```python
from build123d import *

# Parameters (mm, degrees)
SKETCH1_W           = 40
SKETCH1_H           = 40
BOSS_EXTRUDE1_DEPTH = 3
SKETCH2_W           = 40
SKETCH2_H           = 3
BOSS_EXTRUDE2_DEPTH = 53
SKETCH3_W           = 40
SKETCH3_H           = 3
BOSS_EXTRUDE3_DEPTH = 20
CUT_EXTRUDE1_REACH  = 5
FILLET1_R           = 3
SKETCH5_W           = 40
SKETCH5_H           = 3
BOSS_EXTRUDE4_DEPTH = 20


with BuildPart() as part:
    # Sketch1 → Boss-Extrude1 (new body)
    with BuildSketch(Plane(origin=(0, 0, 0), x_dir=(1, 0, 0), z_dir=(0, 1, 0))):
        Rectangle(SKETCH1_W, SKETCH1_H)
    extrude(amount=BOSS_EXTRUDE1_DEPTH)

    # Sketch2 → Boss-Extrude2 (add)
    with BuildSketch(Plane(origin=(0, 0, 0), x_dir=(1, 0, 0), z_dir=(0, 1, 0))):
        with Locations((0, -21.5)):
            Rectangle(SKETCH2_W, SKETCH2_H)
    extrude(amount=BOSS_EXTRUDE2_DEPTH)

    # Sketch3 → Boss-Extrude3 (add)
    with BuildSketch(Plane.XZ):
        with Locations((0, -18.5)):
            Rectangle(SKETCH3_W, SKETCH3_H)
    extrude(amount=BOSS_EXTRUDE3_DEPTH)

    # Sketch4 → Cut-Extrude1 (cut, up to next)
    with BuildSketch(Plane(origin=(0, 0, 20), x_dir=(-1, 0, 0), z_dir=(0, 0, -1)), mode=Mode.PRIVATE) as cut_extrude1_sk1:
        with BuildLine():
            Line((-20, 37.641016151), (-20, 53))
            Line((-20, 53), (20, 53))
            Line((20, 53), (20, 37.641016151))
            ThreePointArc((20, 37.641016151), (0, 43), (-20, 37.641016151))
        make_face()
    cut_extrude1_tool1 = extrude(cut_extrude1_sk1.sketch, amount=-CUT_EXTRUDE1_REACH, mode=Mode.PRIVATE) & part.part
    add(cut_extrude1_tool1.solids().sort_by_distance((0, 47.025808, 20))[0], mode=Mode.SUBTRACT)

    # Fillet1
    fillet1_edges = [part.edges().sort_by_distance(p)[0] for p in [
        (0, 3, 20),
        (0, 3, -20),
    ]]
    fillet(fillet1_edges, radius=FILLET1_R)

    # Sketch5 → Boss-Extrude4 (add)
    with BuildSketch(Plane.XY.offset(-17)):
        with Locations((0, -18.5)):
            Rectangle(SKETCH5_W, SKETCH5_H)
    extrude(amount=BOSS_EXTRUDE4_DEPTH)


solid = part.part
```
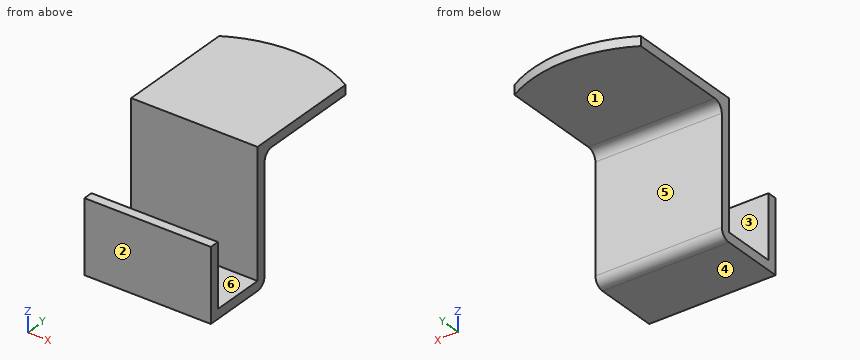
For this review, take the finished solid that the model builds, in its own axes (mm). Face numbers are marked on the shaded views. A direction names the side the tool comes from. Round coordinates to 2 decimals unless told otherwise and drop trailing zeros. Write each loop counter-clockwise with the first axis right and the second up, starting at its lowest first coordinate (ties: lowest second). Pieces come first, ordered by that corner, then holes. Notation, with made-up numbers: (68.25, -28) - (112.25, -28) arc R18 cw to (112.25, -14) - close; hole circle Ø7 at (52, 81.5). An arc over 180 degrees is marked (long way). Answer as CSV lines item,"result". Start each with the question number.
(1) Machinability: for the marked faces 1, 2 and 3, which of the approach directions +Z, -Z, +X, -X, +Y, -Y give a long, thin tool a straight path to every point of the face, cutting with its end or side? Answer none if there is none.
(2) For pin 1 (4 mm diameter, centred on x = 14, z = 12, fed in from +Y); pin 2 (13.5 mm diameter, centred on x = -7, y = -9.5, fed in from +Z); pin 3 (1 mm diameter, centred on x = 1.5, z = 17.5, fed in from -Y); pin 4 (12 mm diameter, centred on y = -4, z = 13, fed in from +X), all flat-tipped, find the tip position at first contact; note any pin that passes through.
(3) Add section A-A, the plane z = -10. State the section outline as (x, y) points.
(4) Add section D-D, the plane x = 7. State the section outline as (y, z) points, plus the area to 3 significant figures.
(5) Mouldability with a two-part tool opening along Y and no side actions: class the marked faces 4, 5 and 6 as +Y half, -Y half, draft (parallel to the pull), parting line (faces both ways), or undercut.
(6) For line 1 (Y direction, x = -9.5, z = 0); line 2 (Z direction, x = -4.5, y = -11); line 3 (Y direction, x = -12, z = 8), list the stretches that pass through material, from the lowest coordinate up.
(7) Add section C-C, the plane y = -11.5. State the section outline as (x, z) points.
(8) Add section B-B, the plane x = 0. State the section outline as (y, z) points, plus the area to 3 significant figures.
From the geometry:
1,face 1,"-Z, +X, -X, +Y"
1,face 2,"+Z, -Z, +X, -X, -Y"
1,face 3,"+Z, +X, -X"
2,pin 1,"stops at y = 3"
2,pin 2,"stops at z = -17"
2,pin 3,"stops at y = 0"
2,pin 4,"stops at x = 20"
3,outline,"(-20, -20) - (20, -20) - (20, -17) - (-20, -17) - close; (-20, 0) - (20, 0) - (20, 3) - (-20, 3) - close"
4,outline,"(-20, -20) - (0, -20) arc R3 ccw to (3, -17) - (3, 17) arc R3 cw to (6, 20) - (42.38, 20) - (42.38, 23) - (0, 23) - (0, -17) - (-17, -17) - (-17, 3) - (-20, 3) - close"
4,area,"367 mm²"
5,face 4,"draft"
5,face 5,"+Y half"
5,face 6,"undercut"
6,line 1,"y = -20 to -17, 0 to 3"
6,line 2,"z = -20 to -17"
6,line 3,"y = 0 to 3"
7,outline,"(-20, -20) - (20, -20) - (20, -17) - (-20, -17) - close"
8,outline,"(-20, -20) - (0, -20) arc R3 ccw to (3, -17) - (3, 17) arc R3 cw to (6, 20) - (43, 20) - (43, 23) - (0, 23) - (0, -17) - (-17, -17) - (-17, 3) - (-20, 3) - close"
8,area,"369 mm²"
